Check sheet for the modelled part. Datum: model origin and axes. Units: mm. Face numbers are marked on the shaded views. A direction names the side the tool comes from. Round coordinates to 2 decimals unless told otherwise and drop trailing zeros. Order: outer loops, then holes, each group sorted by start corner. A loop starts at its lowest first (then second) coordinate and runs counter-clockwise, first axis right, second up.
Q1. Mould release check, pull along X, two halves, no side actions. Record for the marked faces 3, 4, 5 and 6: +X half, -X half, draft (parallel to the pull), parting line (faces both ways), or undercut.
Q2. Cross-section at C-C on x = -3.25. Record the cut outline in (y, z).
Q3. Scan lines: probe 1 along X at (y, z) = (15.5, 1); probe 2 along Z at (x, y) = (-6, 16); probe 3 along Y at (x, z) = (4.5, -13). Record each from-to range of solid material in increasing order.
Q4. Set-up check for the marked faces 1 and 2: record each of +Z, -Z, +X, -X, +Y, -Y from which the full face is reachable in a straight line by a thin tool's end or side.
Q5. Cross-section at A-A on y = 3.25. Record the cut outline in (x, z), then the cut area to 3 significant figures.
Q6. Cross-section at B-B on z = 1.5. Record the cut outline in (x, y).
Q7. Depth check by flat-ended pin: P1, Ø8, axis at x = 1, z = -2.5, coming from the +Y side. Enter the tip coordinate at first touch or a pass-through.
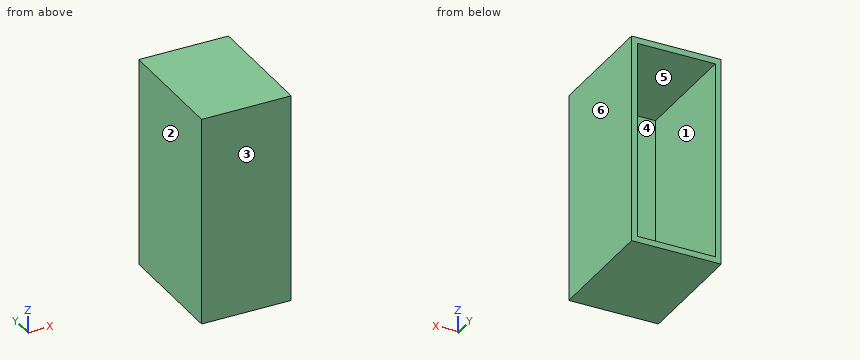
Autodesk Inventor part; units mm, degrees
ref_plane "YZ Plane" through (0, 0, 0) normal (1, 0, 0) x (0, 1, 0)
ref_plane "XZ Plane" through (0, 0, 0) normal (0, 1, 0) x (-1, 0, 0)
ref_plane "XY Plane" through (0, 0, 0) normal (0, 0, 1) x (1, 0, 0)
sketch "Sketch1" plane through (0, 0, 0) normal (0, 1, 0) x (-1, 0, 0)
  line L0 (7.5, 17.5) -> (-7.5, 17.5)
  line L1 (-7.5, 17.5) -> (-7.5, -17.5)
  line L2 (-7.5, -17.5) -> (7.5, -17.5)
  line L3 (7.5, -17.5) -> (7.5, 17.5)
  line L4 (7.5, 17.5) -> (-7.5, -17.5) construction
  line L5 (-7.5, 17.5) -> (7.5, -17.5) construction
  point P0 (0, 0)
  dimension "d0" = 35
  dimension "d1" = 15
extrude "Extrusion1" add sketch "Sketch1" along normal blind 20
shell "Shell1" thickness 1 removed faces 1 at (2.5, 20, -5.8333)
properties part number "servo housing"
Results found:
1. face 3: draft
1. face 4: undercut
1. face 5: undercut
1. face 6: +X half
2. outline: (0, -17.5) - (20, -17.5) - (20, -16.5) - (1, -16.5) - (1, 16.5) - (20, 16.5) - (20, 17.5) - (0, 17.5) - close
3. probe 1: x = -7.5 to -6.5, 6.5 to 7.5
3. probe 2: z = -17.5 to -16.5, 16.5 to 17.5
3. probe 3: y = 0 to 1
4. face 1: +Y
4. face 2: +Z, -Z, -X, +Y, -Y
5. outline: (-7.5, -17.5) - (7.5, -17.5) - (7.5, 17.5) - (-7.5, 17.5) - close; hole (-6.5, -16.5) - (6.5, -16.5) - (6.5, 16.5) - (-6.5, 16.5) - close
5. area: 96.0 mm2
6. outline: (-7.5, 0) - (7.5, 0) - (7.5, 20) - (6.5, 20) - (6.5, 1) - (-6.5, 1) - (-6.5, 20) - (-7.5, 20) - close
7. P1: stops at y = 1
